```python
from build123d import *

# Parameters (mm, degrees)
BOSS_EXTRUDE1_DEPTH = 3
CUT_EXTRUDE2_REACH  = 22.661
SKETCH4_R           = 2.5
BOSS_EXTRUDE4_DEPTH = 3
SKETCH6_R           = 2.5
BOSS_EXTRUDE5_DEPTH = 5


with BuildPart() as part:
    # Sketch1 → Boss-Extrude1 (new body)
    with BuildSketch(Plane(origin=(0, 0, 0), x_dir=(0, 1, 0), z_dir=(0, 0, 1))):
        with BuildLine():
            Line((-16.029850746, -4.082089552), (3.970149254, -4.082089552))
            ThreePointArc((3.970149254, -4.082089552), (7.970149254, -0.082089552), (3.970149254, 3.917910448))
            Line((3.970149254, 3.917910448), (-16.029850746, 3.917910448))
            ThreePointArc((-16.029850746, 3.917910448), (-20.029850746, -0.082089552), (-16.029850746, -4.082089552))
        make_face()
    extrude(amount=BOSS_EXTRUDE1_DEPTH)

    # Sketch4 → Cut-Extrude2 (cut, up to next)
    with BuildSketch(Plane(origin=(0, 0, 3), x_dir=(0, -1, 0), z_dir=(0, 0, 1)), mode=Mode.PRIVATE) as cut_extrude2_sk1:
        with Locations(Location((-3.970149254, 0.082089552, 0), (0, 0, 90))):
            Circle(SKETCH4_R)
    cut_extrude2_tool1 = extrude(cut_extrude2_sk1.sketch, amount=-CUT_EXTRUDE2_REACH, mode=Mode.PRIVATE) & part.part
    add(cut_extrude2_tool1.solids().sort_by_distance((0.08209, 3.970149, 3))[0], mode=Mode.SUBTRACT)

    # Sketch5 → Boss-Extrude4 (add)
    with BuildSketch(Plane.XY.offset(3)):
        Polygon((-0.417910448, 1.470149254), (0.582089552, 1.470149254), (0.132089552, 2.901058056), (0.032089552, 2.901058056), align=None)
        Polygon((-1.60092315, 2.055085744), (-0.734897746, 1.555085744), (-0.409154777, 3.019289117), (-0.495757317, 3.069289117), align=None)
        Polygon((-2.332973957, 3.153161956), (-1.832973957, 2.287136552), (-0.818770584, 3.392302385), (-0.868770584, 3.478904925), align=None)
        Polygon((-2.417910448, 4.470149254), (-2.417910448, 3.470149254), (-0.987001646, 3.920149254), (-0.987001646, 4.020149254), align=None)
        Polygon((-1.832973957, 5.653161956), (-2.332973957, 4.787136552), (-0.868770584, 4.461393582), (-0.818770584, 4.547996123), align=None)
        Polygon((-0.734897746, 6.385212763), (-1.60092315, 5.885212763), (-0.495757317, 4.87100939), (-0.409154777, 4.92100939), align=None)
        Polygon((0.582089552, 6.470149254), (-0.417910448, 6.470149254), (0.032089552, 5.039240452), (0.132089552, 5.039240452), align=None)
        Polygon((1.765102254, 5.885212763), (0.89907685, 6.385212763), (0.573333881, 4.92100939), (0.659936421, 4.87100939), align=None)
        Polygon((2.497153062, 4.787136552), (1.997153062, 5.653161956), (0.982949689, 4.547996123), (1.032949689, 4.461393582), align=None)
        Polygon((2.582089552, 3.470149254), (2.582089552, 4.470149254), (1.15118075, 4.020149254), (1.15118075, 3.920149254), align=None)
        Polygon((1.997153062, 2.287136552), (2.497153062, 3.153161956), (1.032949689, 3.478904925), (0.982949689, 3.392302385), align=None)
        Polygon((0.89907685, 1.555085744), (1.765102254, 2.055085744), (0.659936421, 3.069289117), (0.573333881, 3.019289117), align=None)
    extrude(amount=-BOSS_EXTRUDE4_DEPTH)

    # Sketch6 → Boss-Extrude5 (add)
    with BuildSketch(Plane.XY.offset(3)):
        with Locations((0.082089552, -16.029850746)):
            Circle(SKETCH6_R)
    extrude(amount=BOSS_EXTRUDE5_DEPTH)


solid = part.part
```
The model under review builds one solid part; all positions refer to its coordinate system, in mm. A direction names the side the tool comes from. Round coordinates to 2 decimals unless told otherwise and drop trailing zeros. Loops run counter-clockwise (first coordinate to the right, second up) from the corner with the lowest first, then second, coordinate; pieces in that order, holes last. Notation, with made-up numbers: (-17.5, 52.25) -> (30.5, 52.25) arc R5 cw to (30.5, 59.25) -> close; hole circle Ø7 at (30.5, 50.5). An arc over 180 degrees is marked (long way). Answer in a Markdown table with one row per item.
1) Consider section A-A, the plane z = 5.75. Write out the cut boundary in (x, y).
Taken from the geometry:
| item | result |
|---|---|
| outline | circle Ø5 at (0.08, -16.03) |
2) Consider section B-B, the plane y = -5.25. Write out the cut boundary in (x, z).
Taken from the geometry:
| item | result |
|---|---|
| outline | (-3.92, 0) -> (4.08, 0) -> (4.08, 3) -> (-3.92, 3) -> close |
3) For pin 1 Ø4 at (y, z) = (-5.5, 4.5) entering from -X; pin 2 Ø2.5 at (x, y) = (1.5, 0.5) entering from +Z; pin 3 Ø2 at (x, z) = (2, 6) entering from -Y; pin 4 Ø1 at (x, z) = (3, 2.5) entering from +Y, all flat-tipped, find the tip position at first contact; note any pin that passes through.
Taken from the geometry:
| item | result |
|---|---|
| pin 1 | stops at x = -3.92 |
| pin 2 | stops at z = 3 |
| pin 3 | stops at y = -18.36 |
| pin 4 | stops at y = 7.16 |
4) Tool access review of faces 1 (the flat face through (0, -6, 0)), 2 (the flat face through (-0.564, 5.619, 1.521)), 3 (the cylindrical face through (2.467, -15.279, 5.465)): name each direction out of +Z, -Z, +X, -X, +Y, -Y from which nothing blocks a thin tool from reaching the whole face with its end or side.
Taken from the geometry:
| item | result |
|---|---|
| face 1 | -Z, +X, -X, +Y, -Y |
| face 2 | +Z, -Z |
| face 3 | +Z |
5) Consider section C-C, the plane x = 3.75. Write out the cut boundary in (y, z).
Taken from the geometry:
| item | result |
|---|---|
| outline | (-17.63, 0) -> (5.57, 0) -> (5.57, 3) -> (-17.63, 3) -> close |
6) Consider section D-D, the plane y = -16.75. Write out the cut boundary in (x, z).
Taken from the geometry:
| item | result |
|---|---|
| outline | (-3.85, 0) -> (4.02, 0) -> (4.02, 3) -> (2.48, 3) -> (2.48, 8) -> (-2.31, 8) -> (-2.31, 3) -> (-3.85, 3) -> close |
7) Wall thickness on line 1 along Y through (x, z) = (2.25, 2); line 2 along Z through (x, y) = (-2.5, 0); line 3 along X through (y, z) = (-16.5, 6.5): over which ranges is each line inside the solid? List them lowest first.
Taken from the geometry:
| item | result |
|---|---|
| line 1 | y = -19.39 to 3.21, 3.57 to 4.37, 4.73 to 7.33 |
| line 2 | z = 0 to 3 |
| line 3 | x = -2.37 to 2.54 |
8) Draft analysis for pull direction X (two halves, no side actions). For faces 4 (the flat face through (-1.316, 2.851, 1.521)), 5 (the flat face through (0, -16, 8)), 6 (the flat face through (-3.918, -6, 1)), 7 (the flat face through (1.85, 4.24, 1.52)), state which applies: pulls with the +X half, pulls with the -X half, needs draft (parallel to the pull), parting line crosses it, or undercut.
Taken from the geometry:
| item | result |
|---|---|
| face 4 | undercut |
| face 5 | needs draft |
| face 6 | pulls with the -X half |
| face 7 | undercut |
